Check sheet for the drawn part. Datum: minimum x, y, z corner. Units: mm. A direction names the side the tool comes from. Round coordinates to 2 decimals unless told otherwise and drop trailing zeros. Write each loop counter-clockwise with the first axis right and the second up, starting at its lowest first coordinate (ties: lowest second). Pieces come first, ordered by that corner, then holes. Notation, with made-up numbers: (61.25, -0.75) -> (74.25, -0.75) arc R4 ccw to (74.25, 4.25) -> close; hole circle Ø10 at (11.5, -25). An arc over 180 degrees is marked (long way). One line per item, written item: value. Start each with the question number.
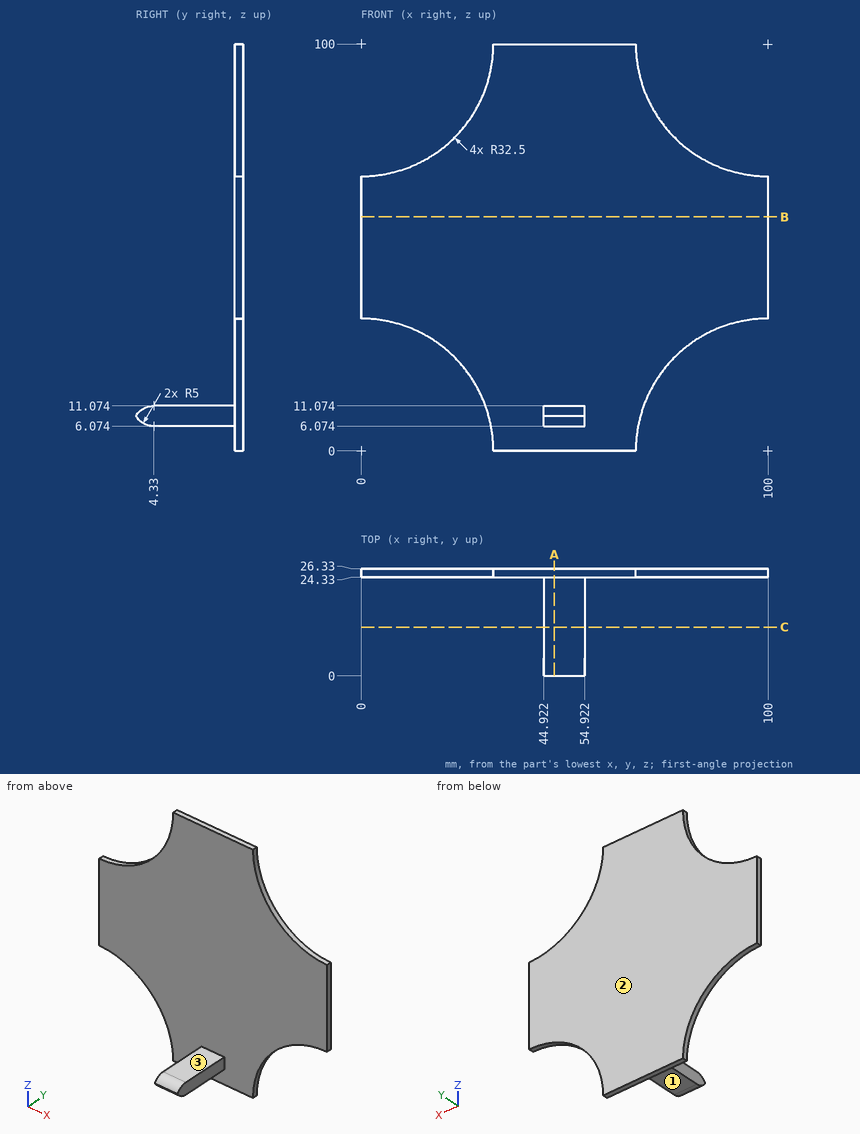
1. Cross-section at A-A (x = 47.5). Record the cut outline in (y, z).
2. Access from +Z, -Z, +X, -X, +Y, -Y to the whole of each face (thin tool, end or side, straight path). Record for the marked faces 1, 2 and 3.
3. Depth check by flat-ended pin: pin 1 Ø8 at (x, y) = (48.5, 10.5) entering from -Z; pin 2 Ø8 at (x, z) = (53, 60.5) entering from -Y; pin 3 Ø2.5 at (y, z) = (8, 8.5) entering from +X. Enter the tip coordinate at first touch or a pass-through.
4. Material ranges on probe 1 along Y at (x, z) = (55, 77.5); probe 2 along Z at (x, y) = (48, 7.75), recorded low to high.
5. Cross-section at C-C (y = 12). Record the cut outline in (x, z), plus the area to 3 significant figures.
6. Cross-section at B-B (z = 57.5). Record the cut outline in (x, y).
Working result:
1. outline: (0, 8.57) arc R5 ccw to (4.33, 6.07) -> (24.33, 6.07) -> (24.33, 0) -> (26.33, 0) -> (26.33, 100) -> (24.33, 100) -> (24.33, 11.07) -> (4.33, 11.07) arc R5 ccw to start
2. face 1: -Z, +X, -X, -Y
2. face 2: +Z, -Z, +X, -X, +Y
2. face 3: +Z, +X, -X, -Y
3. pin 1: stops at z = 6.07
3. pin 2: stops at y = 24.33
3. pin 3: stops at x = 54.92
4. probe 1: y = 24.33 to 26.33
4. probe 2: z = 6.07 to 11.07
5. outline: (44.92, 6.07) -> (54.92, 6.07) -> (54.92, 11.07) -> (44.92, 11.07) -> close
5. area: 50.0 mm^2
6. outline: (0, 24.33) -> (100, 24.33) -> (100, 26.33) -> (0, 26.33) -> close
